```python
from build123d import *

# Parameters (mm, degrees)
SKETCH_R        = 15
PAD_DEPTH       = 6
FILLET_R        = 1
FILLET001_R     = 1
SKETCH001_R     = 12.5
POCKET_DEPTH    = 3
SKETCH002_W     = 20.5
SKETCH002_H     = 6
PAD001_DEPTH    = 25
SKETCH003_R     = 1.55
POCKET001_DEPTH = 20
SKETCH004_R     = 1
POCKET002_DEPTH = 6
FILLET002_R     = 1
FILLET003_R     = 1
FILLET004_R     = 1
FILLET005_R     = 1


with BuildPart() as part:
    # Sketch → Pad (new body)
    with BuildSketch(Plane.XY):
        Circle(SKETCH_R)
    extrude(amount=PAD_DEPTH)

    # Fillet
    fillet_edges = [part.edges().sort_by_distance(p)[0] for p in [
        (-15, 0, 0),
    ]]
    fillet(fillet_edges, radius=FILLET_R)

    # Fillet001
    fillet001_edges = [part.edges().sort_by_distance(p)[0] for p in [
        (-15, 0, 6),
    ]]
    fillet(fillet001_edges, radius=FILLET001_R)

    # Sketch001 (on Face4 of Fillet001) → Pocket (cut)
    with BuildSketch(Plane.XY.offset(6)):
        Circle(SKETCH001_R)
    extrude(amount=-POCKET_DEPTH, mode=Mode.SUBTRACT)

    # Sketch002 (on Face7 of Pocket) → Pad001 (join)
    with BuildSketch(Plane.XY.offset(3)):
        Rectangle(SKETCH002_W, SKETCH002_H)
    extrude(amount=PAD001_DEPTH)

    # Sketch003 (on Face11 of Pad001) → Pocket001 (cut)
    with BuildSketch(Plane(origin=(0, 3, 0), x_dir=(-1, 0, 0), z_dir=(0, 1, 0))):
        with Locations((0, 23)):
            Circle(SKETCH003_R)
        with Locations((0, 15)):
            Circle(SKETCH003_R)
    extrude(amount=-POCKET001_DEPTH, mode=Mode.SUBTRACT)

    # Sketch004 (on Face3 of Pad) → Pocket002 (cut)
    with BuildSketch(Plane.XY.offset(6)):
        with Locations((-5.656854, 5.656854)):
            Circle(SKETCH004_R)
        with Locations((5.656854, 5.656854)):
            Circle(SKETCH004_R)
        with Locations((-5.656854, -5.656854)):
            Circle(SKETCH004_R)
        with Locations((5.656854, -5.656854)):
            Circle(SKETCH004_R)
    extrude(amount=-POCKET002_DEPTH, mode=Mode.SUBTRACT)

    # Fillet002
    fillet002_edges = [part.edges().sort_by_distance(p)[0] for p in [
        (-10.25, -3, 15.5),
    ]]
    fillet(fillet002_edges, radius=FILLET002_R)

    # Fillet003
    fillet003_edges = [part.edges().sort_by_distance(p)[0] for p in [
        (10.25, -3, 15.5),
    ]]
    fillet(fillet003_edges, radius=FILLET003_R)

    # Fillet004
    fillet004_edges = [part.edges().sort_by_distance(p)[0] for p in [
        (10.25, 3, 15.5),
    ]]
    fillet(fillet004_edges, radius=FILLET004_R)

    # Fillet005
    fillet005_edges = [part.edges().sort_by_distance(p)[0] for p in [
        (-10.25, 3, 15.5),
    ]]
    fillet(fillet005_edges, radius=FILLET005_R)


solid = part.part
```
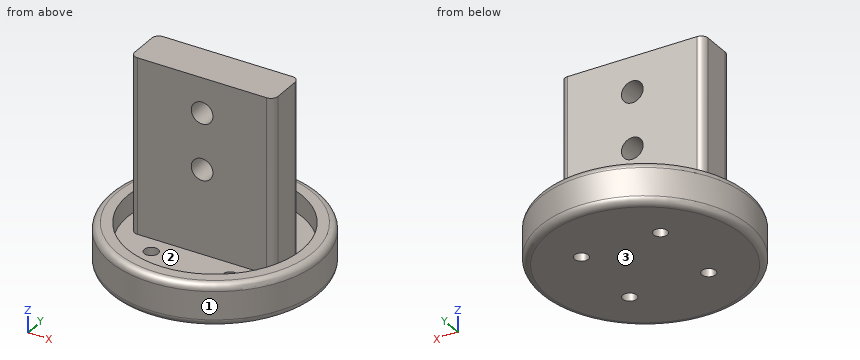
Here's how the part is built. I have some questions about the finished solid (model axes, mm). Face numbers are marked on the shaded views. Coordinates: 2 decimals unless noted, no trailing zeros. Order: outer loops, then holes, each group sorted by start corner. A loop starts at its lowest first (then second) coordinate and runs counter-clockwise, first axis right, second up.
Item 1: If we section it at C-C, the plane x = 0: List the corners of the cut face in (y, z) for me, then the cut area to 3 significant figures.
Response values:
outline: (-15, 1) arc R1 ccw to (-14, 0) - (14, 0) arc R1 ccw to (15, 1) - (15, 5) arc R1 ccw to (14, 6) - (12.5, 6) - (12.5, 3) - (3, 3) - (3, 13.45) - (-3, 13.45) - (-3, 3) - (-12.5, 3) - (-12.5, 6) - (-14, 6) arc R1 ccw to (-15, 5) - close; (-3, 16.55) - (3, 16.55) - (3, 21.45) - (-3, 21.45) - close; (-3, 24.55) - (3, 24.55) - (3, 28) - (-3, 28) - close
area: 217 mm2
Item 2: If we section it at B-B, the plane y = 0: List the corners of the cut face in (x, z) for me, then the cut area to 3 significant figures.
Response values:
outline: (-15, 1) arc R1 ccw to (-14, 0) - (14, 0) arc R1 ccw to (15, 1) - (15, 5) arc R1 ccw to (14, 6) - (12.5, 6) - (12.5, 3) - (10.25, 3) - (10.25, 28) - (-10.25, 28) - (-10.25, 3) - (-12.5, 3) - (-12.5, 6) - (-14, 6) arc R1 ccw to (-15, 5) - close; hole circle Ø3.1 at (0, 15); hole circle Ø3.1 at (0, 23)
area: 602 mm2
Item 3: Thinking about a two-plate mould opening in X: for the marked faces 1, 2 and 3, which applies, pulls with the +X half, pulls with the -X half, needs draft (parallel to the pull), parting line crosses it, or undercut?
Response values:
face 1: parting line crosses it
face 2: undercut
face 3: needs draft
Item 4: I'm going to push flat-ended pins straight in: pin 1 Ø3 at (y, z) = (-3, 23.5) entering from -X; pin 2 Ø5 at (y, z) = (-6.5, 16) entering from +X; pin 3 Ø1 at (x, z) = (6, 10) entering from -Y; pin 4 Ø10 at (x, z) = (5.5, 13) entering from +Y. Where does each tip first touch, or does it pass through?
Response values:
pin 1: stops at x = -10.25
pin 2: passes through
pin 3: stops at y = -3
pin 4: stops at y = 3
Item 5: If we section it at D-D, the plane z = 15: List the corners of the cut face in (x, y) for me, then the cut area to 3 significant figures.
Response values:
outline: (-10.25, -2) arc R1 ccw to (-9.25, -3) - (-1.55, -3) - (-1.55, 3) - (-9.25, 3) arc R1 ccw to (-10.25, 2) - close; (1.55, -3) - (9.25, -3) arc R1 ccw to (10.25, -2) - (10.25, 2) arc R1 ccw to (9.25, 3) - (1.55, 3) - close
area: 104 mm2
Item 6: If we section it at A-A, the plane z = 4.5: List the corners of the cut face in (x, y) for me.
Response values:
outline: circle Ø30 at (0, 0); (-10.25, -2) arc R1 ccw to (-9.25, -3) - (9.25, -3) arc R1 ccw to (10.25, -2) - (10.25, 2) arc R1 ccw to (9.25, 3) - (-9.25, 3) arc R1 ccw to (-10.25, 2) - close; hole circle Ø25 at (0, 0)
Item 7: I need wall thicknesses on probe 1 along Z at (x, y) = (0, -1.55); probe 2 along Y at (x, z) = (-5, 5); probe 3 along Z at (x, y) = (8.5, 3.5). Which ranges of each line are inside material? Lowest first, please.
Response values:
probe 1: z = 0 to 13.45, 16.55 to 21.45, 24.55 to 28
probe 2: y = -14.14 to -11.46, -3 to 3, 11.46 to 14.14
probe 3: z = 0 to 3
